Part model, mm, in its own coordinate system. A direction names the side the tool comes from. Round coordinates to 2 decimals unless told otherwise and drop trailing zeros. Order: outer loops, then holes, each group sorted by start corner. A loop starts at its lowest first (then second) coordinate and runs counter-clockwise, first axis right, second up. Notation, with made-up numbers: (-33, -9.75) - (-17, -9.75) arc R5 cw to (-17, -1.75) - close; hole circle Ø8 at (11.5, -20.75). An arc over 180 degrees is marked (long way). Return JSON: item names as keys, results as strings. Group by question number.
Item 1: Saw through at C-C on y = -2.75. List the corners of the cut face in (x, z).
Item 2: Saw through at D-D on x = -1.5. List the corners of the cut face in (y, z), and give its area (3 significant figures).
Item 3: Probe probe 1 along Z at (x, y) = (-1.5, -2.55); probe 2 along Y at (x, z) = (-1.75, -5); probe 3 along Z at (x, y) = (-0.5, -1). List the from-to ranges inside material, lowest first.
Item 4: Two-plate mould, pull along Z, no slides. Class faces 4 (the face through (3.07, 2.55, -0.05)), 5 (the face through (-0.76, -3.15, 5.58)), 6 (the face through (-1, 1, -3.75)): released by +Z, released by -Z, zero draft, split by the parting line, or undercut.
Item 5: Saw through at A-A on x = 0.75. List the corners of the cut face in (y, z), and give its area (3 significant figures).
Item 6: Saw through at B-B on z = -7. List the corners of the cut face in (x, y), and give its area (3 significant figures).
Item 7: Drop flat-ended pins along their axis: pin 1 (3.5 mm diameter, centred on x = -1, z = -7, fed in from +Y); pin 2 (2 mm diameter, centred on x = -2, y = 0.5, fed in from -Z); pin 3 (2 mm diameter, centred on x = -0.5, y = 2, fed in from +Z). Give the stop position or say it passes through.
Item 8: Tool access for faces 1 (the face through (2.978, -0.905, 7.324)), 2 (the face through (-1, -3, 11)), 3 (the face through (-3, -1.25, -8)): list every direction of +Z, -Z, +X, -X, +Y, -Y with a clear straight run to the whole face (end or side of a thin tool).
```python
from build123d import *

# Parameters (mm, degrees)
F0_W        = 10
F0_H        = 22
F1_DEPTH    = 5
F2_W        = 9.5
F2_H        = 1.25
F3_DEPTH    = 22
F4_R        = 1.5
F5_R        = 1.6
F6_DEPTH    = 3.75
F7_W        = 9.5
F7_H        = 7.5
F8_DEPTH    = 4.25
F9_T1_DEPTH = 10.9475498644
F9_T3_DEPTH = 10.9475498644
F9_T5_DEPTH = 15
F9_T7_DEPTH = 15
F10_R       = 1


# Not quite as in the source:
# - a fillet or chamfer that OpenCascade refuses, or shapes differently, is made with other operations: its cross-section is extruded or revolved along the edge and cut away or added


with BuildPart() as f1:
    # F0 (on Front) → F1 (new body)
    with BuildSketch(Plane.XZ):
        with Locations((-1, 0)):
            Rectangle(F0_W, F0_H)
    extrude(amount=F1_DEPTH)

    # F2 (on face) → F3 (cut, through all)
    with BuildSketch(Plane(origin=(0, 0, -11), x_dir=(1, 0, 0), z_dir=(0, 0, -1))):
        with Locations((-1.25, 0.625)):
            Rectangle(F2_W, F2_H)
    extrude(amount=-F3_DEPTH, mode=Mode.SUBTRACT)

    # F4
    f4_edges = [f1.edges().sort_by_distance(p)[0] for p in [
        (4, -5, 0),
    ]]
    fillet(f4_edges, radius=F4_R)

    # F5 (on face) → F6 (cut, through all)
    with BuildSketch(Plane.XZ.offset(5)):
        with Locations((-1.5, 7)):
            Circle(F5_R)
        with Locations((-1.5, -7)):
            Circle(F5_R)
    extrude(amount=-F6_DEPTH, mode=Mode.SUBTRACT)

    # F7 (on face) → F8 (join)
    with BuildSketch(Plane(origin=(0, -1.25, 0), x_dir=(-1, 0, 0), z_dir=(0, 1, 0))):
        with Locations((1.25, 0)):
            Rectangle(F7_W, F7_H)
    extrude(amount=F8_DEPTH)

    # F9: fillet of radius 1.5 on 4 edges, made by hand

    # F9_s2 → F9_t1 (join)
    with BuildSketch(Plane.XY.offset(0.0524501356)):
        with BuildLine():
            ThreePointArc((2.0209800542, -1.25), (2.9892258908, -0.8956439237), (3.5, 0))
            Line((3.5, 0), (3.5, -1.25))
            Line((3.5, -1.25), (2.0209800542, -1.25))
        make_face()
    extrude(amount=F9_T1_DEPTH)

    # F9_s4 → F9_t3 (join)
    with BuildSketch(Plane.XY.offset(-11)):
        with BuildLine():
            ThreePointArc((2.0209800542, -1.25), (2.9892258908, -0.8956439237), (3.5, 0))
            Line((3.5, 0), (3.5, -1.25))
            Line((3.5, -1.25), (2.0209800542, -1.25))
        make_face()
    extrude(amount=F9_T3_DEPTH)

    # F9_s6 → F9_t5 (cut)
    with BuildSketch(Plane.XY.offset(-7.5)):
        with BuildLine():
            ThreePointArc((-4.5, 3), (-5.5606601718, 2.5606601718), (-6, 1.5))
            Line((-6, 1.5), (-6, 3))
            Line((-6, 3), (-4.5, 3))
        make_face()
    extrude(amount=F9_T5_DEPTH, mode=Mode.SUBTRACT)

    # F9_s8 → F9_t7 (cut)
    with BuildSketch(Plane.XY.offset(-7.5)):
        with BuildLine():
            ThreePointArc((3.5, 1.5), (3.0606601718, 2.5606601718), (2, 3))
            Line((2, 3), (3.5, 3))
            Line((3.5, 3), (3.5, 1.5))
        make_face()
    extrude(amount=F9_T7_DEPTH, mode=Mode.SUBTRACT)

    # F10
    f10_edges = [f1.edges().sort_by_distance(p)[0] for p in [
        (-6, -5, 0),
    ]]
    fillet(f10_edges, radius=F10_R)


solid = f1.part
```
Filled in:
{
 "1": {"outline": "(-6, -11) - (4, -11) - (4, 11) - (-6, 11) - close; hole circle Ø3.2 at (-1.5, -7); hole circle Ø3.2 at (-1.5, 7)"},
 "2": {"outline": "(-5, -11) - (-1.25, -11) - (-1.25, -8.6) - (-5, -8.6) - close; (-5, -5.4) - (-1.25, -5.4) - (-1.25, -3.75) - (3, -3.75) - (3, 3.75) - (-1.25, 3.75) - (-1.25, 5.4) - (-5, 5.4) - close; (-5, 8.6) - (-1.25, 8.6) - (-1.25, 11) - (-5, 11) - close", "area": "90.4 mm^2"},
 "3": {"probe 1": "z = -11 to -8.6, -5.4 to 5.4, 8.6 to 11", "probe 2": "y = -5 to -1.25", "probe 3": "z = -3.75 to 3.75"},
 "4": {"face 4": "zero draft", "face 5": "undercut", "face 6": "released by -Z"},
 "5": {"outline": "(-5, -11) - (-1.25, -11) - (-1.25, -3.75) - (3, -3.75) - (3, 3.75) - (-1.25, 3.75) - (-1.25, 11) - (-5, 11) - close", "area": "114 mm^2"},
 "6": {"outline": "(-6, -4) arc R1 ccw to (-5, -5) - (-3.1, -5) - (-3.1, -1.25) - (-6, -1.25) - close; (0.1, -5) - (2.5, -5) arc R1.5 ccw to (4, -3.5) - (4, 0) - (3.5, 0) arc R1.5 cw to (2.02, -1.25) - (0.1, -1.25) - close", "area": "25.9 mm^2"},
 "7": {"pin 1": "stops at y = -1.25", "pin 2": "stops at z = -3.75", "pin 3": "stops at z = 3.75"},
 "8": {"face 1": "+Z, -X, +Y", "face 2": "+Z, +X, -X, +Y, -Y", "face 3": "-Z, -X, +Y"}
}
